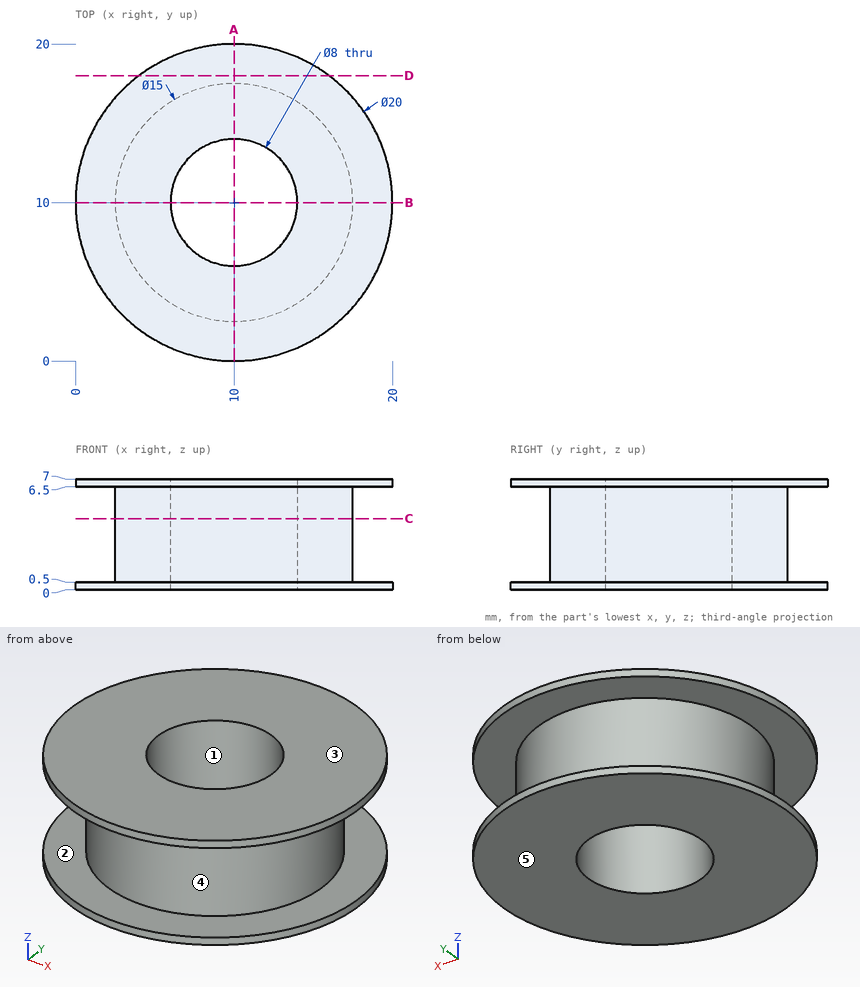
Geometry check sheet. Reference: drawing and pictorial views, mm from the part's lowest x, y, z. A direction names the side the tool comes from. Coordinates: 2 decimals unless noted, no trailing zeros. Write each loop counter-clockwise with the first axis right and the second up, starting at its lowest first coordinate (ties: lowest second). Pieces come first, ordered by that corner, then holes. Notation, with made-up numbers: (-27, -1) - (-1, -1) arc R21 cw to (-1, 20) - close; hole circle Ø5 at (-24.5, 43). An arc over 180 degrees is marked (long way). One line per question, with ' | ' between items. Start each with the question number.
1. Gauge pin test, flat ends, axial feed: P1, Ø1.5, axis at y = 8, z = 5.5, coming from the +X side; P2, Ø1.5, axis at y = 5, z = 5.5, coming from the +X side. Record the tip position at first contact, or that the pin passes through.
2. Draft check along Z on the marked faces 1, 2 and 3. Enter one of: released by +Z, released by -Z, zero draft, split by the parting line, or undercut.
3. Section check D-D (y = 18). Enter the section's corners in (x, z).
4. Material ranges on line 1 along Z through (x, y) = (14.25, 3.75); line 2 along Y through (x, z) = (10, 2.5); line 3 along X through (y, z) = (7.5, 1.5), recorded low to high.
5. Section check C-C (z = 4.5). Enter the section's corners in (x, y).
6. Access from +Z, -Z, +X, -X, +Y, -Y to the whole of each face (thin tool, end or side, straight path). Record for the marked faces 4 and 5.
7. Section check A-A (x = 10). Enter the section's corners in (y, z).
Computed values:
1) P1: x = 17.4 | P2: x = 16.18
2) face 1: zero draft | face 2: undercut | face 3: released by +Z
3) outline: (4, 0) - (16, 0) - (16, 0.5) - (4, 0.5) - close; (4, 6.5) - (16, 6.5) - (16, 7) - (4, 7) - close
4) line 1: 0 to 0.5, 6.5 to 7 | line 2: 2.5 to 6, 14 to 17.5 | line 3: 2.93 to 6.88, 13.12 to 17.07
5) outline: circle Ø15 at (10, 10); hole circle Ø8 at (10, 10)
6) face 4: none | face 5: -Z, +X, -X, +Y, -Y
7) outline: (0, 0) - (6, 0) - (6, 7) - (0, 7) - (0, 6.5) - (2.5, 6.5) - (2.5, 0.5) - (0, 0.5) - close; (14, 0) - (20, 0) - (20, 0.5) - (17.5, 0.5) - (17.5, 6.5) - (20, 6.5) - (20, 7) - (14, 7) - close
